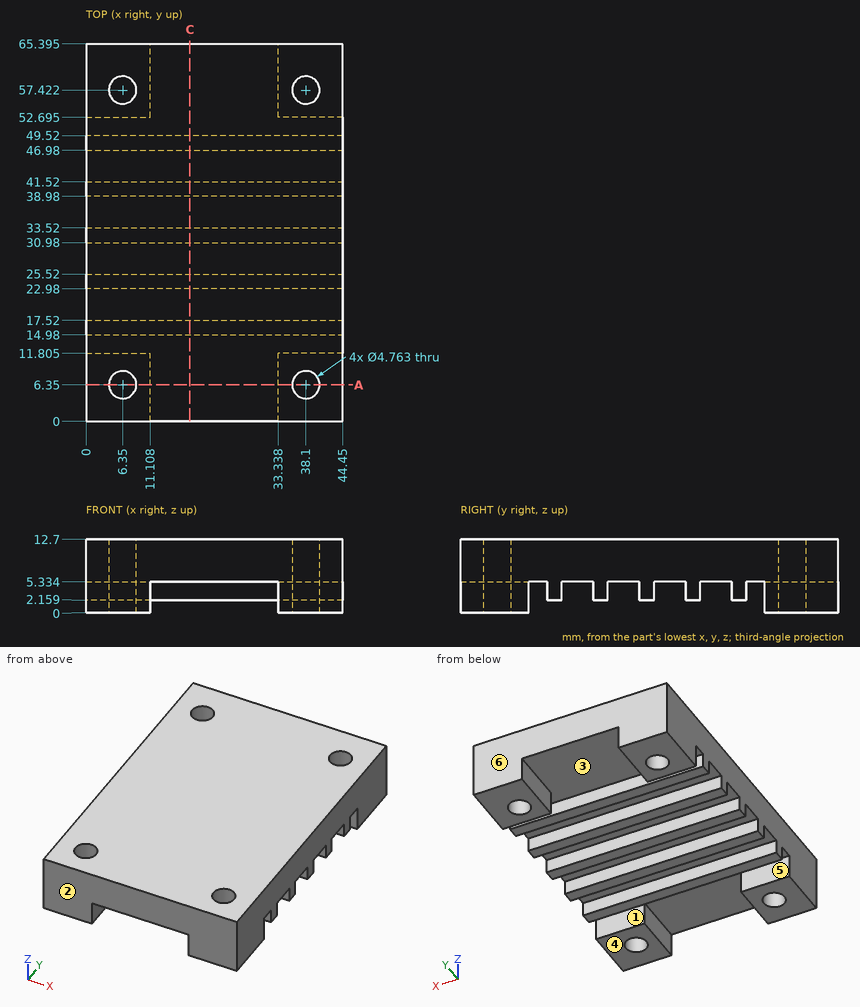
Job drawing, mm, ordinate dimensions from the low corner. One solid piece. A direction names the side the tool comes from. Round coordinates to 2 decimals unless told otherwise and drop trailing zeros. Loops run counter-clockwise (first coordinate to the right, second up) from the corner with the lowest first, then second, coordinate; pieces in that order, holes last.
Item 1: Mould opens along Y. For the marked faces 1, 2, 3 and 4 say: +Y half, -Y half, draft (parallel to the pull), parting line (faces both ways), or undercut.
Item 2: Cut at A-A, the plane y = 6.35. State how many separate pieces and enclosed holes the cut face has, then the cut area to 3 significant figures.
Item 3: Cut at C-C, the plane x = 18. Give the cut face in (y, z) (1 decimal), then the cut area to 3 significant figures.
Item 4: Drop flat-ended pins along their axis: P1, Ø3, axis at x = 33.5, y = 41.5, coming from the -Z side; P2, Ø4.5, axis at x = 18, y = 9, coming from the -Z side; P3, Ø2, axis at x = 16.5, z = 2.5, coming from the +Y side. Give the stop position or say it passes through.
Item 5: 3-axis set-ups, long thin cutter, end or side, ignore diameter. For the marked faces 5 and 6: which of +Z, -Z, +X, -X, +Y, -Y reach the whole face in a straight line?
Item 6: Drill centre lines: line 1 (Y direction, x = 6.35, z = 10.25) (1 decimal); line 2 (Y direction, x = 15, z = 4.25); line 3 (Y direction, x = 34.5, z = 1.5) (1 decimal). Where is each one in solid material? Low to high.
A:
1. face 1: undercut
1. face 2: -Y half
1. face 3: undercut
1. face 4: draft
2. separate pieces: 3
2. enclosed holes: 0
2. area: 325 mm2
3. outline: (0, 5.3) - (15, 5.3) - (15, 2.2) - (17.5, 2.2) - (17.5, 5.3) - (23, 5.3) - (23, 2.2) - (25.5, 2.2) - (25.5, 5.3) - (31, 5.3) - (31, 2.2) - (33.5, 2.2) - (33.5, 5.3) - (39, 5.3) - (39, 2.2) - (41.5, 2.2) - (41.5, 5.3) - (47, 5.3) - (47, 2.2) - (49.5, 2.2) - (49.5, 5.3) - (65.4, 5.3) - (65.4, 12.7) - (0, 12.7) - close
3. area: 522 mm2
4. P1: stops at z = 2.16
4. P2: stops at z = 5.33
4. P3: stops at y = 49.52
5. face 5: -Z, +X, -X
5. face 6: +Z, -Z, +X, -X, +Y
6. line 1: y = 0 to 4, 8.7 to 55, 59.8 to 65.4
6. line 2: y = 14.98 to 17.52, 22.98 to 25.52, 30.98 to 33.52, 38.98 to 41.52, 46.98 to 49.52
6. line 3: y = 0 to 11.8, 52.7 to 65.4
